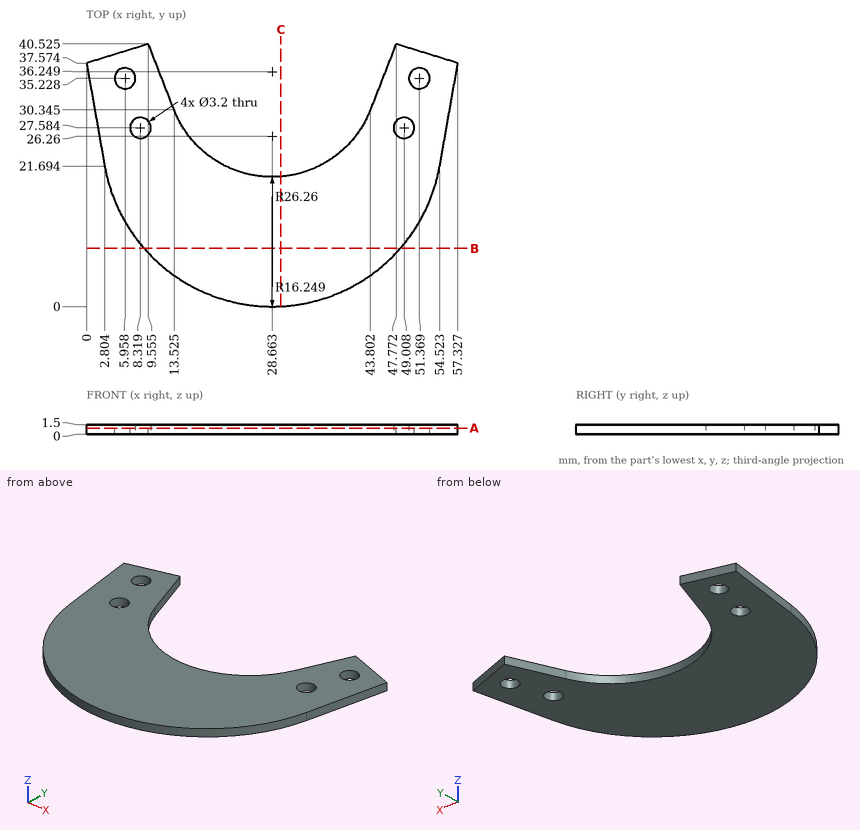
Print and shaded views of the part. All mm, measured from the part's lowest x, y and z. Round coordinates to 2 decimals unless told otherwise and drop trailing zeros. Write each loop counter-clockwise with the first axis right and the second up, starting at its lowest first coordinate (ties: lowest second). Pieces come first, ordered by that corner, then holes. Notation, with made-up numbers: (-36, 51.5) -> (-27, 51.5) arc R8 ccw to (-27, 66.5) -> close; hole circle Ø2 at (6, -26.5). An arc over 180 degrees is marked (long way). Answer in a Markdown table with one row per item. Add a question column.
Item 1: Saw through at C-C, the plane x = 30. Write the cut outline in (y, z) (1 decimal).
Item 2: Drop flat-ended pins along their axis: pin 1 Ø2.5 at (x, y) = (49.01, 27.58) entering from -Z (1 decimal); pin 2 Ø2 at (x, y) = (40.5, 7.5) entering from -Z. Give the stop position or say it passes through.
Item 3: Drill centre lines: line 1 (X direction, y = 35, z = 0.85) (1 decimal); line 2 (X direction, y = 34, z = 0.4) (1 decimal); line 3 (X direction, y = 18, z = 0.85). Where is each one in solid material? Low to high. Write a range as from..to.
Item 4: Saw through at B-B, the plane y = 9. Write the cut outline in (x, z).
Item 5: Saw through at A-A, the plane z = 0.95. Write the cut outline in (x, y) (1 decimal), then the cut area to 3 significant figures.
Findings below:
| question | item | result |
|---|---|---|
| 1 | outline | (0, 0) -> (20.1, 0) -> (20.1, 1.5) -> (0, 1.5) -> close |
| 2 | pin 1 | passes through |
| 2 | pin 2 | stops at z = 0 |
| 3 | line 1 | x = 0.5..4.4, 7.5..11.7, 45.6..49.8, 53..56.9 |
| 3 | line 2 | x = 0.6..4.9, 7..12.1, 45.2..50.3, 52.4..56.7 |
| 3 | line 3 | x = 3.74..53.59 |
| 4 | outline | (8.87, 0) -> (48.45, 0) -> (48.45, 1.5) -> (8.87, 1.5) -> close |
| 5 | outline | (0, 37.6) -> (2.8, 21.7) arc R26.3 ccw to (54.5, 21.7) -> (57.3, 37.6) -> (47.8, 40.5) -> (43.8, 30.3) arc R16.2 cw to (13.5, 30.3) -> (9.6, 40.5) -> close; hole circle Ø3.2 at (6, 35.2); hole circle Ø3.2 at (8.3, 27.6); hole circle Ø3.2 at (49, 27.6); hole circle Ø3.2 at (51.4, 35.2) |
| 5 | area | 1,240 mm^2 |
